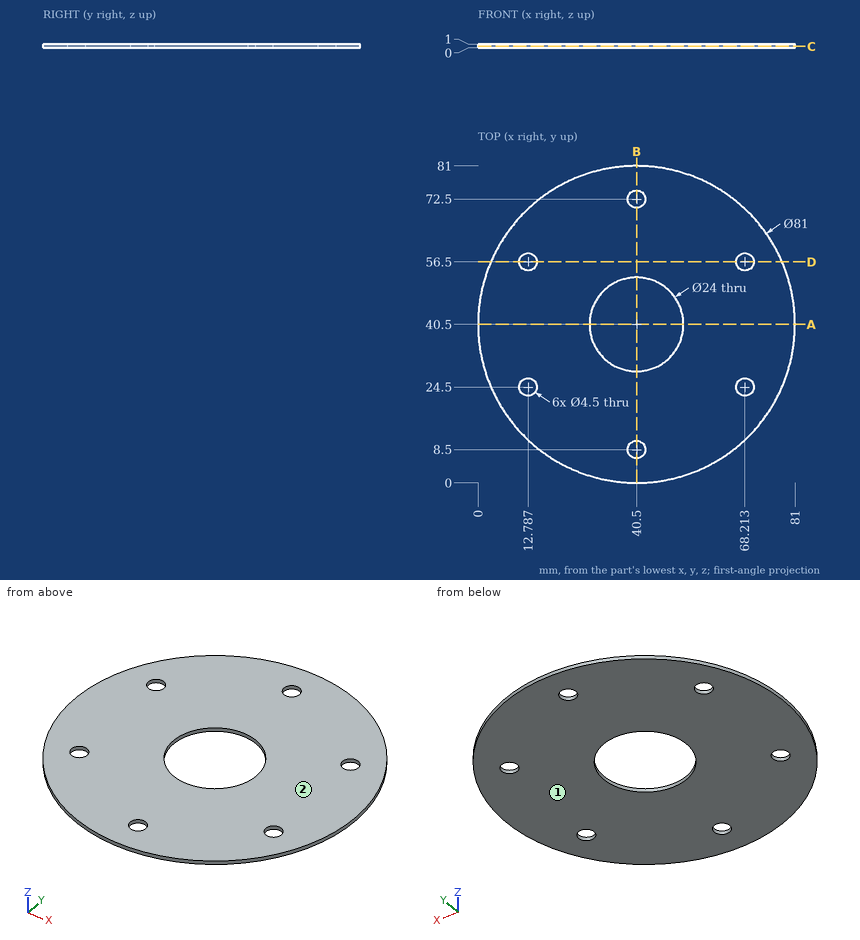
The figure shows three views and two pictorial views of one solid part (mm, origin at its lowest corner). Answer the questions. Give positions to 0.01 mm unless a question says otherwise; leave off trailing zeros. Loops run counter-clockwise (first coordinate to the right, second up) from the corner with the lowest first, then second, coordinate; pieces in that order, holes last. Notation, with made-up numbers: (42.25, 66.5) -> (61.25, 66.5) arc R27 cw to (61.25, 89.5) -> close; hole circle Ø5 at (-11.5, -5). An arc over 180 degrees is marked (long way). Use a Markdown table: item, result. Add a question column.
1. Section B-B on x = 40.5 is taken. Determine the outline of the cut face in (y, z).
2. Section D-D on y = 56.5 is taken. Determine the outline of the cut face in (x, z).
3. Find the intervals of material crossed by probe 1 along Y at (x, z) = (40.5, 0.55); probe 2 along X at (y, z) = (24.5, 0.8) (1 decimal); probe 3 along X at (y, z) = (25, 0.9), in increasing order.
4. Determine the mould class of the marked faces 1 and 2 for opening direction Z: released by +Z, released by -Z, zero draft, split by the parting line, or undercut.
5. Section C-C on z = 0.4 is taken. Determine the outline of the cut face in (x, y).
6. Section A-A on y = 40.5 is taken. Determine the outline of the cut face in (x, z).
7. A flat-ended cylindrical pin translates along its axis: pin 1 Ø2.5 at (x, y) = (68.21, 56.5) entering from +Z. Find the tip coordinate at first contact, or state that the pin passes through.
Results below:
| question | item | result |
|---|---|---|
| 1 | outline | (0, 0) -> (6.25, 0) -> (6.25, 1) -> (0, 1) -> close; (10.75, 0) -> (28.5, 0) -> (28.5, 1) -> (10.75, 1) -> close; (52.5, 0) -> (70.25, 0) -> (70.25, 1) -> (52.5, 1) -> close; (74.75, 0) -> (81, 0) -> (81, 1) -> (74.75, 1) -> close |
| 2 | outline | (3.29, 0) -> (10.54, 0) -> (10.54, 1) -> (3.29, 1) -> close; (15.04, 0) -> (65.96, 0) -> (65.96, 1) -> (15.04, 1) -> close; (70.46, 0) -> (77.71, 0) -> (77.71, 1) -> (70.46, 1) -> close |
| 3 | probe 1 | y = 0 to 6.25, 10.75 to 28.5, 52.5 to 70.25, 74.75 to 81 |
| 3 | probe 2 | x = 3.3 to 10.5, 15 to 66, 70.5 to 77.7 |
| 3 | probe 3 | x = 3.08 to 10.59, 14.98 to 66.02, 70.41 to 77.92 |
| 4 | face 1 | released by -Z |
| 4 | face 2 | released by +Z |
| 5 | outline | circle Ø81 at (40.5, 40.5); hole circle Ø4.5 at (12.79, 24.5); hole circle Ø4.5 at (12.79, 56.5); hole circle Ø24 at (40.5, 40.5); hole circle Ø4.5 at (40.5, 8.5); hole circle Ø4.5 at (40.5, 72.5); hole circle Ø4.5 at (68.21, 24.5); hole circle Ø4.5 at (68.21, 56.5) |
| 6 | outline | (0, 0) -> (28.5, 0) -> (28.5, 1) -> (0, 1) -> close; (52.5, 0) -> (81, 0) -> (81, 1) -> (52.5, 1) -> close |
| 7 | pin 1 | passes through |
